from build123d import *

# Parameters (mm, degrees)
SHAFT_D_FLAT_DEPTH      = 55.733353634
SHAFT_D_FLAT_DEPTH_BACK = 55.733353634
SKETCH2_W               = 1.5
SKETCH2_H               = 8.5
SKETCH3_R               = 1.25
M3_MOUNTING_HOLES_DEPTH = 3.5


with BuildPart() as part:
    # Sketch1 → Motor Body (revolve)
    with BuildSketch(Plane(origin=(0, 0, 0), x_dir=(-1, 0, 0), z_dir=(0, 1, 0)), mode=Mode.PRIVATE) as motor_body_sk:
        Polygon((0, 11.5), (-2, 11.5), (-2, 2.5), (-3.5, 2.5), (-3.5, 0), (-12.5, 0), (-12.5, -21), (-12.2, -21), (-12.2, -51.8), (0, -51.8), align=None)
    revolve(motor_body_sk.sketch.rotate(Axis((0, 0, -60), (0, 0, 1)), 180), axis=Axis((0, 0, -60), (0, 0, 1)))

    # Sketch2 → Shaft D-Flat (cut, two sides: drawn at the far end of the back side and taken through both)
    with BuildSketch(Plane(origin=(0, 0, 0), x_dir=(-1, 0, 0), z_dir=(0, 1, 0)).offset(-SHAFT_D_FLAT_DEPTH_BACK)):
        with Locations((-2.25, 7.75)):
            Rectangle(SKETCH2_W, SKETCH2_H)
    extrude(amount=SHAFT_D_FLAT_DEPTH + SHAFT_D_FLAT_DEPTH_BACK, mode=Mode.SUBTRACT)

    # Sketch3 → M3 Mounting Holes (cut)
    with BuildSketch(Plane(origin=(0, 0, 0), x_dir=(0, 1, 0), z_dir=(0, 0, 1))):
        with Locations(Location((4.875399709, -6.962792376, 0), (0, 0, 270))):
            Circle(SKETCH3_R)
        with Locations(Location((-4.875399709, 6.962792376, 0), (0, 0, 270))):
            Circle(SKETCH3_R)
    extrude(amount=-M3_MOUNTING_HOLES_DEPTH, mode=Mode.SUBTRACT)


solid = part.part
CAD build for the part. Positions are in the model's coordinates, mm. A direction names the side the tool comes from. Give positions to 0.01 mm unless a question says otherwise; leave off trailing zeros. Order: outer loops, then holes, each group sorted by start corner. A loop starts at its lowest first (then second) coordinate and runs counter-clockwise, first axis right, second up. Notation, with made-up numbers: (73, 66) - (128, 66) arc R22 cw to (128, 81) - close; hole circle Ø1 at (58.5, -28). An arc over 180 degrees is marked (long way). Answer in a Markdown table with one row per item.
1. Saw through at B-B, the plane x = 0. Give the cut face in (y, z), plus the area to 3 significant figures.
Data:
| item | result |
|---|---|
| outline | (-12.5, -21) - (-12.2, -21) - (-12.2, -51.8) - (12.2, -51.8) - (12.2, -21) - (12.5, -21) - (12.5, 0) - (3.5, 0) - (3.5, 2.5) - (2, 2.5) - (2, 11.5) - (-2, 11.5) - (-2, 2.5) - (-3.5, 2.5) - (-3.5, 0) - (-12.5, 0) - close |
| area | 1,330 mm² |
2. Probe probe 1 along Z at (x, y) = (-1, -6.75); probe 2 along Z at (x, y) = (2.25, -2); probe 3 along X at (y, z) = (-10.75, -1). List the from-to ranges inside material, lowest first. Write a range as [from, to].
Data:
| item | result |
|---|---|
| probe 1 | z = [-51.8, 0] |
| probe 2 | z = [-51.8, 2.5] |
| probe 3 | x = [-6.38, 6.38] |
3. Tool access for faces 1 (the cylindrical face through (12.19, -0.54, -36.62)), 2 (the flat face through (2, 2, 2.5)), 3 (the flat face through (0, 0, 11.5)), 4 (the flat face through (1.5, 0, 7)), 5 (the flat face through (0, 0, -51.8)): list every direction of +Z, -Z, +X, -X, +Y, -Y with a clear straight run to the whole face (end or side of a thin tool).
Data:
| item | result |
|---|---|
| face 1 | -Z |
| face 2 | +Z |
| face 3 | +Z, +X, -X, +Y, -Y |
| face 4 | +Z, +X, +Y, -Y |
| face 5 | -Z, +X, -X, +Y, -Y |
4. Pull direction X, two halves, no side cores. Call faces 6 (the flat face through (-7, -5, -3.5)), 7 (the flat face through (3, 3, 0)), 8 (the cylindrical face through (-1.908, -0.601, 6.937)), 9 (the flat face through (7, 5, -3.5)): pulls with the +X half, pulls with the -X half, needs draft (parallel to the pull), parting line crosses it, or undercut.
Data:
| item | result |
|---|---|
| face 6 | undercut |
| face 7 | needs draft |
| face 8 | parting line crosses it |
| face 9 | undercut |
5. Saw through at D-D, the plane z = -2. Give the cut face in (x, y), plus the area to 3 significant figures.
Data:
| item | result |
|---|---|
| outline | circle Ø25 at (0, 0); hole circle Ø2.5 at (-6.96, -4.88); hole circle Ø2.5 at (6.96, 4.88) |
| area | 481 mm² |
6. Saw through at A-A, the plane y = 0. Give the cut face in (x, z).
Data:
| item | result |
|---|---|
| outline | (-12.5, -21) - (-12.2, -21) - (-12.2, -51.8) - (12.2, -51.8) - (12.2, -21) - (12.5, -21) - (12.5, 0) - (3.5, 0) - (3.5, 2.5) - (2, 2.5) - (2, 3.5) - (1.5, 3.5) - (1.5, 11.5) - (-2, 11.5) - (-2, 2.5) - (-3.5, 2.5) - (-3.5, 0) - (-12.5, 0) - close |
7. Flat gauge pins, fed straight in: pin 1 (2 mm diameter, centred on x = 7, y = 4.5, fed in from +Z); pin 2 (5 mm diameter, centred on y = -7, z = -0.5, fed in from -X); pin 3 (1.5 mm diameter, centred on y = 5, z = -31, fed in from -X). Where does each tip first touch, or does it go through?
Data:
| item | result |
|---|---|
| pin 1 | stops at z = 0 |
| pin 2 | stops at x = -11.66 |
| pin 3 | stops at x = -11.44 |
8. Saw through at C-C, the plane z = 6. Give the cut face in (x, y).
Data:
| item | result |
|---|---|
| outline | (1.5, -1.32) - (1.5, 1.32) arc R2 ccw (long way) to start |
